Verification items for the finished model (mm, model axes). A direction names the side the tool comes from. Round coordinates to 2 decimals unless told otherwise and drop trailing zeros. Order: outer loops, then holes, each group sorted by start corner. A loop starts at its lowest first (then second) coordinate and runs counter-clockwise, first axis right, second up. Notation, with made-up numbers: (66, -36) -> (91, -36) arc R16 cw to (91, -9) -> close; hole circle Ø7 at (29, 66). An arc over 180 degrees is marked (long way). Answer in a Markdown table with one row per item. Add a question column.
```python
from build123d import *

# Parameters (mm, degrees)
F0_W      = 15.96
F0_H      = 8.3576925244
F1_DEPTH  = 32.5
F2_W      = 15.9
F2_H      = 6.4
F3_DEPTH  = 15.5
F4_DEPTH  = 70
F6_DEPTH  = 25
F7_R      = 2.45
F8_DEPTH  = 2
F7_W      = 15.9
F7_H      = 7.8
F8_FACE_R = 2.45
F9_DEPTH  = 1.5
F10_R     = 2.45
F10_R_2   = 1.55
F11_DEPTH = 5.9
F12_R     = 2.45
F12_R_2   = 1.55
F13_DEPTH = 1.9
F14_DEPTH = 4
F15_DEPTH = 4
F16_W     = 14.4657706842
F16_H     = 5.8139935136
F16_R     = 2.228006958
F17_DEPTH = 2
F19_DEPTH = 12.5


with BuildPart() as f1:
    # F0 (on Front) → F1 (new body)
    with BuildSketch(Plane.XZ):
        Polygon((15.9, 3.1903535793), (-15.9, 3.1903535793), (-15.9, -6.5096464207), (-6.726923441, -6.5096464207), (-6.726923441, 1.8480461037), (9.233076559, 1.8480461037), (9.233076559, -6.5096464207), (15.9, -6.5096464207), align=None)
        with Locations((1.253076559, -2.3308001585)):
            Rectangle(F0_W, F0_H)
    extrude(amount=F1_DEPTH)

    # F2 (on face) → F3 (cut)
    with BuildSketch(Plane.XZ.offset(32.5)):
        with Locations((0, -3.3096464207)):
            Rectangle(F2_W, F2_H)
    extrude(amount=-F3_DEPTH, mode=Mode.SUBTRACT)

    # F2 (on face) → F4 (cut)
    with BuildSketch(Plane.XZ.offset(32.5)):
        Polygon((-15.9, 3.1903535793), (-15.9, -6.3096464207), (-8.1, 3.1903535793), align=None)
        Polygon((8.1, 3.1903535793), (15.9, -6.3096464207), (15.9, 3.1903535793), align=None)
    extrude(amount=-F4_DEPTH, mode=Mode.SUBTRACT)

    # F5 (on face) → F6 (cut)
    with BuildSketch(Plane(origin=(0, 0, -6.5096464207), x_dir=(1, 0, 0), z_dir=(0, 0, -1))):
        Polygon((-8, 0), (-15.9, 24.7), (-15.9, 0), align=None)
        Polygon((15.9, 24.7), (8, 0), (15.9, 0), align=None)
    extrude(amount=-F6_DEPTH, mode=Mode.SUBTRACT)

    # F7 (on face) → F8 (join)
    with BuildSketch(Plane(origin=(0, 0, -0.1096464207), x_dir=(1, 0, 0), z_dir=(0, 0, -1))):
        with Locations((-4.0132352151, 28.5375677049)):
            Circle(F7_R)
        with Locations((4.0132352151, 28.5375677049)):
            Circle(F7_R)
    extrude(amount=F8_DEPTH)

    # F7 (on face) + F1_face1 (on face) + F8_face (on face) → F9 (join)
    with BuildSketch(Plane(origin=(0, 0, -0.1096464207), x_dir=(1, 0, 0), z_dir=(0, 0, -1))):
        with Locations((0, 28.6)):
            Rectangle(F7_W, F7_H)
        with Locations((-4.0132352151, 28.5375677049)):
            Circle(F7_R, mode=Mode.SUBTRACT)
        with Locations((4.0132352151, 28.5375677049)):
            Circle(F7_R, mode=Mode.SUBTRACT)
    with BuildSketch(Plane(origin=(0, -13.5883838384, -6.5096464207), x_dir=(1, 0, 0), z_dir=(0, 0, -1))):
        Polygon((-8, -13.5883838384), (8, -13.5883838384), (15.9, 11.1116161616), (15.9, 18.9116161616), (7.95, 18.9116161616), (7.95, 3.4116161616), (-7.95, 3.4116161616), (-7.95, 18.9116161616), (-15.9, 18.9116161616), (-15.9, 11.1116161616), align=None)
    with BuildSketch(Plane(origin=(-4.0132352151, -28.5375677049, -2.1096464207), x_dir=(1, 0, 0), z_dir=(0, 0, -1))):
        Circle(F8_FACE_R)
        with Locations((8.0264704302, 0)):
            Circle(F8_FACE_R)
    extrude(amount=F9_DEPTH)

    # F10 (on face) → F11 (join)
    with BuildSketch(Plane(origin=(0, 0, -0.1096464207), x_dir=(1, 0, 0), z_dir=(0, 0, -1))):
        with Locations((-3.7897760311, 20.9340956062)):
            Circle(F10_R)
        with Locations((-3.7897760311, 20.9340956062)):
            Circle(F10_R_2, mode=Mode.SUBTRACT)
        with Locations((3.8324711446, 20.9340956062)):
            Circle(F10_R)
        with Locations((3.8324711446, 20.9340956062)):
            Circle(F10_R_2, mode=Mode.SUBTRACT)
    extrude(amount=F11_DEPTH)

    # F12 (on face) → F13 (join)
    with BuildSketch(Plane(origin=(0, 0, -8.0096464207), x_dir=(1, 0, 0), z_dir=(0, 0, -1))):
        with Locations((-11.9673879817, 29.0735326707)):
            Circle(F12_R)
        with Locations((-11.9673879817, 29.0735326707)):
            Circle(F12_R_2, mode=Mode.SUBTRACT)
        with Locations((11.9673879817, 29.0735326707)):
            Circle(F12_R)
        with Locations((11.9673879817, 29.0735326707)):
            Circle(F12_R_2, mode=Mode.SUBTRACT)
    extrude(amount=F13_DEPTH)

    # F12 (on face) → F14 (join)
    with BuildSketch(Plane(origin=(0, 0, -8.0096464207), x_dir=(1, 0, 0), z_dir=(0, 0, -1))):
        with Locations((-4.5118764974, 12.756055221)):
            Circle(F12_R)
        with Locations((-4.5118764974, 12.756055221)):
            Circle(F12_R_2, mode=Mode.SUBTRACT)
        with Locations((4.5118764974, 12.756055221)):
            Circle(F12_R)
        with Locations((4.5118764974, 12.756055221)):
            Circle(F12_R_2, mode=Mode.SUBTRACT)
    extrude(amount=F14_DEPTH)

    # F12 (on face) → F15 (join)
    with BuildSketch(Plane(origin=(0, 0, -8.0096464207), x_dir=(1, 0, 0), z_dir=(0, 0, -1))):
        with Locations((-4.7830846161, 5.5871135555)):
            Circle(F12_R)
        with Locations((-4.7830846161, 5.5871135555)):
            Circle(F12_R_2, mode=Mode.SUBTRACT)
        with Locations((4.7830846161, 5.5871135555)):
            Circle(F12_R)
        with Locations((4.7830846161, 5.5871135555)):
            Circle(F12_R_2, mode=Mode.SUBTRACT)
    extrude(amount=F15_DEPTH)

    # F16 (on face) → F17 (cut)
    with BuildSketch(Plane.XY.offset(3.1903535793)):
        with Locations((-0.0129453838, -28.7997983396)):
            Rectangle(F16_W, F16_H)
        with Locations((0, -28.9382264018)):
            Circle(F16_R, mode=Mode.SUBTRACT)
    extrude(amount=-F17_DEPTH, mode=Mode.SUBTRACT)

    # F18 (on Right) → F19 (cut, symmetric)
    with BuildSketch(Plane.YZ):
        Polygon((-25.8897673339, 3.1903535793), (0, -6.7096464207), (0, 3.1903535793), (-0.3126582278, 3.1903535793), align=None)
    extrude(amount=F19_DEPTH, both=True, mode=Mode.SUBTRACT)


solid = f1.part
```
1) Cross-section at A-A, the plane z = -4.5. Record the boundary of the cut face in (x, y).
2) Cross-section at D-D, the plane z = -1. Record the boundary of the cut face in (x, y).
3) Draft check along X on faces 4 (the face through (-7.95, -25, -4)), 5 (the face through (-11.9, -12.2, -5.6)), 6 (the face through (0, -29, 3.19)). Enter one of: +X half, -X half, draft (parallel to the pull), parting line (faces both ways), or undercut.
4) Tool access check on faces 1 (the face through (-7.246, -29, 2)), 2 (the face through (6.4, -6.2, -12.01)), 3 (the face through (3.482, -26.146, -2.596)). Record the directions out of +Z, -Z, +X, -X, +Y, -Y that give a thin tool (end or side, any length) a straight path to the whole face; none if there is none.
5) Cross-section at C-C, the plane z = 2. Record the boundary of the cut face in (x, y), and give its area (3 significant figures).
6) Depth check by flat-ended pin: P1, Ø4, axis at x = -3.79, y = -20.93, coming from the -Z side; P2, Ø5, axis at y = -26.5, z = -1, coming from the -X side; P3, Ø2.5, axis at x = 4.78, y = -5.59, coming from the +Z side; P4, Ø1.5, axis at x = -12, z = 0, coming from the +Y side. Enter the tip coordinate at first touch or a pass-through.
7) Thickness scan on L1, parallel to X at y = -30, z = 1.5; L2, parallel to Z at x = 7, y = -29.5; L3, parallel to Z at x = -4, y = -30.5. Record the ranges inside material, lowest first. Write a range as [from, to].
Results below:
| question | item | result |
|---|---|---|
| 1 | outline | (-14.41, -32.5) -> (-7.95, -32.5) -> (-7.95, -17) -> (7.95, -17) -> (7.95, -32.5) -> (14.41, -32.5) -> (14.41, -20.05) -> (9.85, -5.78) -> (-9.85, -5.78) -> (-14.41, -20.05) -> close; circle Ø4.9 at (-3.79, -20.93); circle Ø4.9 at (3.83, -20.93); hole circle Ø3.1 at (-3.79, -20.93); hole circle Ø3.1 at (3.83, -20.93) |
| 2 | outline | (-11.54, -32.5) -> (11.54, -32.5) -> (11.54, -14.93) -> (-11.54, -14.93) -> close; circle Ø4.9 at (-3.79, -20.93); circle Ø4.9 at (3.83, -20.93); hole (-7.95, -24.7) -> (7.95, -24.7) -> (7.95, -17) -> (-7.95, -17) -> close; hole circle Ø3.1 at (-3.79, -20.93); hole circle Ø3.1 at (3.83, -20.93) |
| 3 | face 4 | undercut |
| 3 | face 5 | -X half |
| 3 | face 6 | draft |
| 4 | face 1 | +Z |
| 4 | face 2 | -Z, +X, -X, +Y, -Y |
| 4 | face 3 | -Z |
| 5 | outline | (-9.08, -32.5) -> (9.08, -32.5) -> (9.08, -22.78) -> (-9.08, -22.78) -> close; circle Ø4.46 at (0, -28.94); hole (-7.25, -31.71) -> (7.22, -31.71) -> (7.22, -25.89) -> (-7.25, -25.89) -> close |
| 5 | area | 108 mm² |
| 6 | P1 | z = -6.01 |
| 6 | P2 | x = -13.59 |
| 6 | P3 | z = -4.09 |
| 6 | P4 | through |
| 7 | L1 | [-9.49, -7.25], [-1.96, 1.96], [7.22, 9.49] |
| 7 | L2 | [-1.61, 1.19] |
| 7 | L3 | [-3.61, 1.19] |
